Geometry: see drawing. Coordinates: mm, zero at the bounding-box minimum. A direction names the side the tool comes from. Give positions to 0.01 mm unless a question says otherwise; leave off trailing zeros. Write each loop counter-clockwise with the first axis right and the second up, starting at its lowest first coordinate (ties: lowest second). Pieces come first, ordered by that corner, then holes. Notation, with made-up numbers: (52, -18.75) - (98, -18.75) arc R25 ccw to (98, -3.75) - close; hole circle Ø6 at (56, 69). An arc over 180 degrees is marked (long way). One line per question, with ' | ' between items. Start each with the question number.
(1) Access query for the marked faces 1 and 2. Directions: +Z, -Z, +X, -X, +Y, -Y. A direction counts if a zero-diameter tool reaches every point of the face in a straight line with its end or side. Return the directions, or none.
(2) Ray query, line 1 (X direction, y = 7.5, z = 5.5); line 2 (Y direction, x = 22.5, z = 6); line 3 (X direction, y = 6.25, z = 7.5). Return the intervals inside material, ascending. Write a range as [from, to].
(3) Section C-C, the plane z = 9.5. Return loops of the section in (x, y).
(4) Section A-A, the plane x = 22.5. Return loops of the section in (y, z).
(5) Section D-D, the plane x = 15.25. Return loops of the section in (y, z), plus the area to 3 significant figures.
(6) Section B-B, the plane y = 7.5. Return loops of the section in (x, z), plus the area to 3 significant figures.
(7) Pin query (flat end, axial travel): pin 1 (8 mm diameter, centred on x = 7.5, y = 10, fed in from -Z); pin 2 (0.8 mm diameter, centred on x = 11.5, y = 14, fed in from +Z); pin 3 (0.6 mm diameter, centred on x = 12, z = 9, fed in from +Y). Return the tip coordinate at first contact, or that it passes through.
(8) Draft query along Y for the marked faces 3, 4 and 5. Return one class per face: +Y half, -Y half, draft (parallel to the pull), parting line (faces both ways), or undercut.
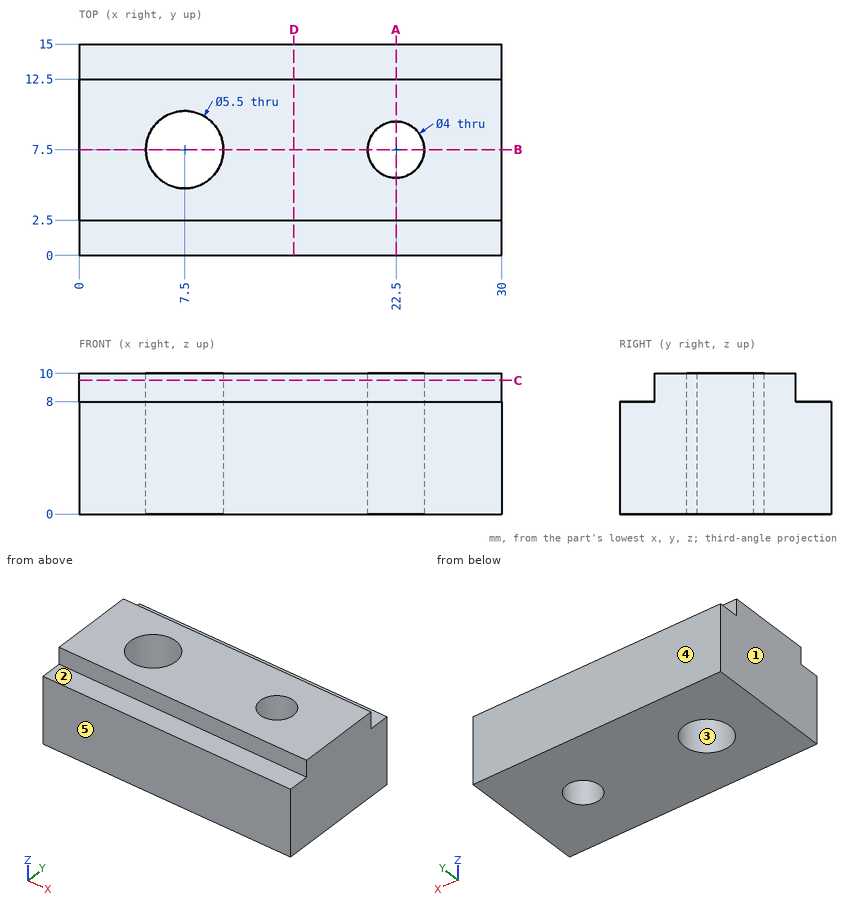
Check sheet entries:
1) face 1: +Z, -Z, -X, +Y, -Y | face 2: +Z, +X, -X, -Y
2) line 1: [0, 4.75], [10.25, 20.5], [24.5, 30] | line 2: [0, 5.5], [9.5, 15] | line 3: [0, 5.05], [9.95, 20.94], [24.06, 30]
3) outline: (0, 2.5) - (30, 2.5) - (30, 12.5) - (0, 12.5) - close; hole circle Ø5.5 at (7.5, 7.5); hole circle Ø4 at (22.5, 7.5)
4) outline: (0, 0) - (5.5, 0) - (5.5, 10) - (2.5, 10) - (2.5, 8) - (0, 8) - close; (9.5, 0) - (15, 0) - (15, 8) - (12.5, 8) - (12.5, 10) - (9.5, 10) - close
5) outline: (0, 0) - (15, 0) - (15, 8) - (12.5, 8) - (12.5, 10) - (2.5, 10) - (2.5, 8) - (0, 8) - close | area: 140 mm²
6) outline: (0, 0) - (4.75, 0) - (4.75, 10) - (0, 10) - close; (10.25, 0) - (20.5, 0) - (20.5, 10) - (10.25, 10) - close; (24.5, 0) - (30, 0) - (30, 10) - (24.5, 10) - close | area: 205 mm²
7) pin 1: z = 0 | pin 2: z = 8 | pin 3: y = 12.5
8) face 3: undercut | face 4: +Y half | face 5: -Y half
